Source: CAD feature listing. Evaluate the final solid. Frame: model axes, mm. Coordinates: 2 decimals unless noted, no trailing zeros. Order: outer loops, then holes, each group sorted by start corner. A loop starts at its lowest first (then second) coordinate and runs counter-clockwise, first axis right, second up.
```python
from build123d import *

# Parameters (mm, degrees)
F0_R     = 2.8769537575
F1_DEPTH = 25.4


with BuildPart() as f1:
    # F0 (on Top) → F1 (new body)
    with BuildSketch(Plane.XY):
        Polygon((0, 52.07), (0, 0), (25.4, 0), (25.4, 104.14), (0, 104.14), align=None)
        with Locations((5.715, 12.065)):
            Circle(F0_R, mode=Mode.SUBTRACT)
        with BuildLine():
            ThreePointArc((14.2875, 5.08), (11.5774679849, 3.9574679849), (12.7, 6.6675))
            ThreePointArc((12.7, 6.6675), (13.8225320151, 6.2025320151), (14.2875, 5.08))
        make_face(mode=Mode.SUBTRACT)
        with Locations((5.715, 29.845)):
            Circle(F0_R, mode=Mode.SUBTRACT)
        with BuildLine():
            ThreePointArc((8.5919537575, 47.625), (2.9527786647, 46.820639249), (8.1421750872, 49.1695659646))
            ThreePointArc((8.1421750872, 49.1695659646), (8.4772213353, 48.429360751), (8.5919537575, 47.625))
        make_face(mode=Mode.SUBTRACT)
        with Locations((19.685, 20.955)):
            Circle(F0_R, mode=Mode.SUBTRACT)
        with Locations((19.685, 38.735)):
            Circle(F0_R, mode=Mode.SUBTRACT)
        with BuildLine():
            ThreePointArc((8.5919537575, 65.405), (8.4772213353, 64.600639249), (8.1421750872, 63.8604340354))
            ThreePointArc((8.1421750872, 63.8604340354), (2.9527786647, 66.209360751), (8.5919537575, 65.405))
        make_face(mode=Mode.SUBTRACT)
        with Locations((5.715, 83.185)):
            Circle(F0_R, mode=Mode.SUBTRACT)
        with BuildLine():
            ThreePointArc((14.2875, 99.06), (13.8225320151, 97.9374679849), (12.7, 97.4725))
            ThreePointArc((12.7, 97.4725), (11.5774679849, 100.1825320151), (14.2875, 99.06))
        make_face(mode=Mode.SUBTRACT)
        with BuildLine():
            Line((17.2578249128, 54.9704340354), (12.7, 52.07))
            Line((12.7, 52.07), (12.7, 60.96))
            Line((12.7, 60.96), (17.2578249128, 58.0595659646))
            ThreePointArc((17.2578249128, 58.0595659646), (20.489360751, 59.2772213353), (22.5619537575, 56.515))
            ThreePointArc((22.5619537575, 56.515), (20.489360751, 53.7527786647), (17.2578249128, 54.9704340354))
        make_face(mode=Mode.SUBTRACT)
        with Locations((19.685, 74.295)):
            Circle(F0_R, mode=Mode.SUBTRACT)
        with Locations((19.685, 92.075)):
            Circle(F0_R, mode=Mode.SUBTRACT)
        with BuildLine():
            Line((12.7, 60.96), (12.7, 52.07))
            Line((12.7, 52.07), (17.2578249128, 54.9704340354))
            ThreePointArc((17.2578249128, 54.9704340354), (16.8080462425, 56.515), (17.2578249128, 58.0595659646))
            Line((17.2578249128, 58.0595659646), (12.7, 60.96))
        make_face()
    extrude(amount=F1_DEPTH)


solid = f1.part
```
Q1. Section query B-B on z = 11.5. Give the number of separate pieces and of enclosed holes in the cut face, plus the area to 3 significant figures.
Solutions:
separate pieces: 1
enclosed holes: 12
area: 2,370 mm2
Q2. Material intervals for line 1 along Y through (x, z) = (12.5, 2); line 2 along X through (y, z) = (21, 4); line 3 along Y through (x, z) = (8.25, 13.25), sorted ascending.
Solutions:
line 1: y = 0 to 3.51, 6.65 to 97.49, 100.63 to 104.14
line 2: x = 0 to 16.81, 22.56 to 25.4
line 3: y = 0 to 10.7, 13.43 to 28.48, 31.21 to 46.26, 48.99 to 64.04, 66.77 to 81.82, 84.55 to 104.14
Q3. Section query C-C on x = 18.5. Output: boundary loops of the cut face in (y, z).
Solutions:
outline: (0, 0) - (18.33, 0) - (18.33, 25.4) - (0, 25.4) - close; (23.58, 0) - (36.11, 0) - (36.11, 25.4) - (23.58, 25.4) - close; (41.36, 0) - (53.89, 0) - (53.89, 25.4) - (41.36, 25.4) - close; (59.14, 0) - (71.67, 0) - (71.67, 25.4) - (59.14, 25.4) - close; (76.92, 0) - (89.45, 0) - (89.45, 25.4) - (76.92, 25.4) - close; (94.7, 0) - (104.14, 0) - (104.14, 25.4) - (94.7, 25.4) - close
Q4. Pin query (flat end, axial travel): P1, Ø5, axis at x = 5.715, y = 47.625, coming from the +Z side. Return the tip coordinate at first contact, or that it passes through.
Solutions:
P1: passes through
Q5. Pull-direction query (X, two-part tool) for faces 1 (the flat face through (13, 0, 13)), 2 (the flat face through (0, 53, 13)), 3 (the flat face through (25.4, 51, 13)), 4 (the cylindrical face through (22.43, 21.82, 12.52)); classes: pulls with the +X half, pulls with the -X half, needs draft (parallel to the pull), parting line crosses it, or undercut.
Solutions:
face 1: needs draft
face 2: pulls with the -X half
face 3: pulls with the +X half
face 4: undercut
Q6. Section query A-A on y = 66.5. Output: boundary loops of the cut face in (x, z), plus the area to 3 significant figures.
Solutions:
outline: (0, 0) - (3.05, 0) - (3.05, 25.4) - (0, 25.4) - close; (8.38, 0) - (25.4, 0) - (25.4, 25.4) - (8.38, 25.4) - close
area: 510 mm2
